```python
from build123d import *

# Parameters (mm, degrees)
BOSS_EXTRUDE1_DEPTH                        = 157.1625
F_10_32_TAPPED_HOLE1_D                     = 4.0386
F_10_32_TAPPED_HOLE1_DEPTH                 = 16.764
F_10_32_TAPPED_HOLE1_CBORE_D               = 4.826
F_10_32_TAPPED_HOLE1_CBORE_DEPTH           = 12.7
F_10_32_TAPPED_HOLE1_TIP                   = 1.213317848
F_10_32_TAPPED_HOLE1_ON_FACE_2_D           = 4.0386
F_10_32_TAPPED_HOLE1_ON_FACE_2_DEPTH       = 16.764
F_10_32_TAPPED_HOLE1_ON_FACE_2_CBORE_D     = 4.826
F_10_32_TAPPED_HOLE1_ON_FACE_2_CBORE_DEPTH = 12.7
F_10_32_TAPPED_HOLE1_ON_FACE_2_TIP         = 1.213317848


with BuildPart() as part:
    # Sketch1 → Boss-Extrude1 (new body)
    with BuildSketch(Plane(origin=(0, 0, 0), x_dir=(1, 0, 0), z_dir=(0, 1, 0))):
        Polygon((0, 7.332348419), (-6.35, 3.666174209), (-6.35, -3.666174209), (0, -7.332348419), (6.35, -3.666174209), (6.35, 3.666174209), align=None)
    extrude(amount=BOSS_EXTRUDE1_DEPTH)

    # #10-32 Tapped Hole1
    with Locations(Plane.ZX.offset(157.1625)):
        with Locations((0, 0)):
            CounterBoreHole(F_10_32_TAPPED_HOLE1_D / 2, F_10_32_TAPPED_HOLE1_CBORE_D / 2, F_10_32_TAPPED_HOLE1_CBORE_DEPTH, depth=F_10_32_TAPPED_HOLE1_DEPTH)
            with Locations((0, 0, -(F_10_32_TAPPED_HOLE1_DEPTH + F_10_32_TAPPED_HOLE1_TIP / 2))):  # 118° drill point
                Cone(0, F_10_32_TAPPED_HOLE1_D / 2, F_10_32_TAPPED_HOLE1_TIP, mode=Mode.SUBTRACT)

    # #10-32 Tapped Hole1 on face 2
    with Locations(Plane(origin=(0, 0, 0), x_dir=(0, 0, -1), z_dir=(0, -1, 0))):
        with Locations((0, 0)):
            CounterBoreHole(F_10_32_TAPPED_HOLE1_ON_FACE_2_D / 2, F_10_32_TAPPED_HOLE1_ON_FACE_2_CBORE_D / 2, F_10_32_TAPPED_HOLE1_ON_FACE_2_CBORE_DEPTH, depth=F_10_32_TAPPED_HOLE1_ON_FACE_2_DEPTH)
            with Locations((0, 0, -(F_10_32_TAPPED_HOLE1_ON_FACE_2_DEPTH + F_10_32_TAPPED_HOLE1_ON_FACE_2_TIP / 2))):  # 118° drill point
                Cone(0, F_10_32_TAPPED_HOLE1_ON_FACE_2_D / 2, F_10_32_TAPPED_HOLE1_ON_FACE_2_TIP, mode=Mode.SUBTRACT)


solid = part.part
```
The listing builds one solid part. Answer for the finished solid, in the listing's coordinates (mm). A direction names the side the tool comes from. Give positions to 0.01 mm unless a question says otherwise; leave off trailing zeros. Loops run counter-clockwise (first coordinate to the right, second up) from the corner with the lowest first, then second, coordinate; pieces in that order, holes last. Notation, with made-up numbers: M 87.25,37 L 104.25,37 A21 ccw 104.25,75 Z; hole C -19,72.25 d6. An arc over 180 degrees is marked long. One line per item, written item: value.
Q1. Determine the mould class of faces 1 (the face through (6.35, 77, 0)), 2 (the face through (0.607, 142.402, -1.926)), 3 (the face through (3.219, 77.481, -5.474)) for opening direction Z: +Z half, -Z half, draft (parallel to the pull), parting line (faces both ways), or undercut.
Working result:
face 1: draft
face 2: undercut
face 3: -Z half
Q2. For faces 4 (the face through (-1.468, 6.261, 1.915)), 5 (the face through (-3.131, 77.481, -5.525)), 6 (the face through (-2, 144.462, -1)), determine the directions among +Z, -Z, +X, -X, +Y, -Y from which every point of the face is accessible in a straight line to the end or side of a thin tool.
Working result:
face 4: -Y
face 5: -Z, -X, +Y, -Y
face 6: +Y
Q3. Find the intervals of material crossed by line 1 (X direction, y = 142.4, z = 0); line 2 (X direction, y = 149, z = 0); line 3 (Z direction, x = -1.75, y = 76.5), in increasing order. Write a range as from..to.
Working result:
line 1: x = -6.35..-2.02, 2.02..6.35
line 2: x = -6.35..-2.41, 2.41..6.35
line 3: z = -6.32..6.32
Q4. Flat-ended cylindrical pins translate along their axes: P1, Ø4.5, axis at x = 0, z = 0, coming from the +Y side; P2, Ø7.5, axis at x = 0, z = 0, coming from the +Y side; P3, Ø3.5, axis at x = 0, z = 0, coming from the -Y side; P4, Ø3, axis at x = 0, z = 0, coming from the +Y side. Find the tip coordinate at first contact, or state that the pin passes through.
Working result:
P1: stops at y = 144.46
P2: stops at y = 157.16
P3: stops at y = 16.93
P4: stops at y = 140.09
Q5. A cutting plane is placed at A-A on x = 4.5. Determine the outline of the cut face in (y, z).
Working result:
outline: M 0,-4.73 L 157.16,-4.73 L 157.16,4.73 L 0,4.73 Z
